```python
from build123d import *

# Parameters (mm, degrees)
EXTRUDE_START     = -5
SKETCH_1_W        = 62.97
SKETCH_1_H        = 62.97
SKETCH_1_W_2      = 60.97
SKETCH_1_H_2      = 60.97
EXTRUDE_1_DEPTH   = 14
SKETCH_3_W        = 62.97
SKETCH_3_H        = 62.97
EXTRUDE_1_2_DEPTH = 1


with BuildPart() as part:
    # 草图1 → Extrude 1 (new body)
    with BuildSketch(Plane.XY.offset(EXTRUDE_START)):
        with Locations((29.873059436, -30.254060198)):
            Rectangle(SKETCH_1_W, SKETCH_1_H)
        with Locations((29.873059436, -30.254060198)):
            Rectangle(SKETCH_1_W_2, SKETCH_1_H_2, mode=Mode.SUBTRACT)
    extrude(amount=EXTRUDE_1_DEPTH)

    # 草图3 → Extrude 1 2 (add)
    with BuildSketch(Plane(origin=(0, 0, -5), x_dir=(-1, 0, 0), z_dir=(0, 0, -1))):
        with Locations((-29.873059436, -30.254060198)):
            Rectangle(SKETCH_3_W, SKETCH_3_H)
    extrude(amount=EXTRUDE_1_2_DEPTH)


solid = part.part
```
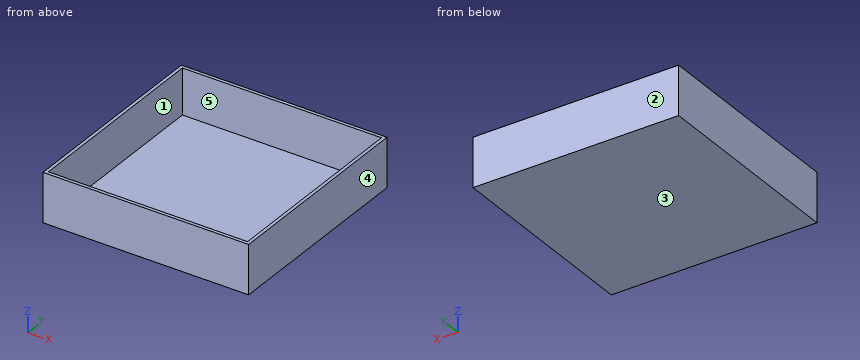
Can you work these out from the model? Positions are in its coordinate system, mm. Face numbers are marked on the shaded views. A direction names the side the tool comes from. Coordinates: 2 decimals unless noted, no trailing zeros. Loops run counter-clockwise (first coordinate to the right, second up) from the corner with the lowest first, then second, coordinate; pieces in that order, holes last.
1) Imagine slicing it at C-C on y = -23.5. List the corners of the cut face in (x, z) for me, plus the area to 3 significant figures.
2) I need wall thicknesses on probe 1 along X at (y, z) = (-20, 0.75); probe 2 along Y at (x, z) = (29.5, 3.5); probe 3 along Z at (x, y) = (7, -44). Which ranges of each line are inside material? Lowest first, please.
3) For pin 1 (2 mm diameter, centred on x = 52.5, y = -22, fed in from +Z), with a flat end and sliding along its axis, tell me the tip position at first contact or that it passes through.
4) Which directions (+Z, -Z, +X, -X, +Y, -Y) give clear straight access to the entire face, cutting with the end or side of a thin tool? Please do the marked faces 4 and 5.
5) Imagine slicing it at A-A on z = -3.75. List the corners of the cut face in (x, y) for me.
6) Thinking about a two-plate mould opening in Y: for the marked faces 1, 2 and 3, which applies, pulls with the +Y half, pulls with the -Y half, needs draft (parallel to the pull), parting line crosses it, or undercut?
7) Imagine slicing it at B-B on x = 15.5. List the corners of the cut face in (y, z) for me, plus the area to 3 significant figures.
Completed:
1. outline: (-1.61, -6) - (61.36, -6) - (61.36, 9) - (60.36, 9) - (60.36, -5) - (-0.61, -5) - (-0.61, 9) - (-1.61, 9) - close
1. area: 91.0 mm2
2. probe 1: x = -1.61 to -0.61, 60.36 to 61.36
2. probe 2: y = -61.74 to -60.74, 0.23 to 1.23
2. probe 3: z = -6 to -5
3. pin 1: stops at z = -5
4. face 4: +Z, -Z, +X, +Y, -Y
4. face 5: +Z
5. outline: (-1.61, -61.74) - (61.36, -61.74) - (61.36, 1.23) - (-1.61, 1.23) - close; hole (-0.61, -60.74) - (60.36, -60.74) - (60.36, 0.23) - (-0.61, 0.23) - close
6. face 1: undercut
6. face 2: pulls with the +Y half
6. face 3: needs draft
7. outline: (-61.74, -6) - (1.23, -6) - (1.23, 9) - (0.23, 9) - (0.23, -5) - (-60.74, -5) - (-60.74, 9) - (-61.74, 9) - close
7. area: 91.0 mm2
